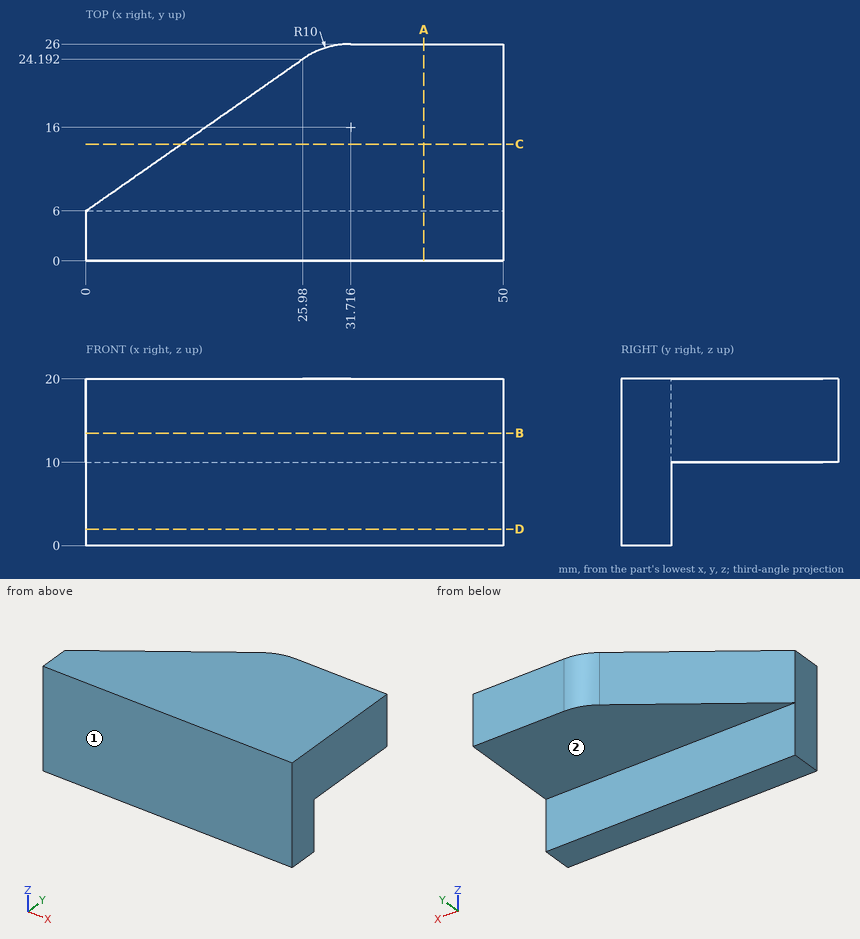
Input: dimensioned drawing with shaded views. Units: mm. Origin: part minimum x, y, z. A direction names the side the tool comes from. Coordinates: 2 decimals unless noted, no trailing zeros. Loops run counter-clockwise (first coordinate to the right, second up) from the corner with the lowest first, then second, coordinate; pieces in that order, holes last.
Q1. Set-up query: the marked faces 1 and 2. Return all of +Z, -Z, +X, -X, +Y, -Y with unobstructed straight access to the full face (end or side cutting, diameter ignored); none if empty.
Results are:
face 1: +Z, -Z, +X, -X, -Y
face 2: -Z, +X, -X, +Y
Q2. Section A-A, the plane x = 40.5. Return the cut outline in (y, z), and give its area (3 significant figures).
Results are:
outline: (0, 0) - (6, 0) - (6, 10) - (26, 10) - (26, 20) - (0, 20) - close
area: 320 mm2
Q3. Contact query for a flat-ended pin moving along its axis: pin 1 (1.5 mm diameter, centred on x = 15.5, z = 8, fed in from +Y). Output: stop coordinate, or through.
Results are:
pin 1: stops at y = 6
Q4. Line query: line 1 along Y through (x, z) = (43, 5.25); line 2 along Z through (x, y) = (19.5, 14.25); line 3 along X through (y, z) = (19.5, 10.5). Output: solid intervals per line, ascending.
Results are:
line 1: y = 0 to 6
line 2: z = 10 to 20
line 3: x = 19.28 to 50
Q5. Section D-D, the plane z = 2. Return the cut outline in (x, y), and give its area (3 significant figures).
Results are:
outline: (0, 0) - (50, 0) - (50, 6) - (0, 6) - close
area: 300 mm2
Q6. Section B-B, the plane z = 13.5. Return the cut outline in (x, y) (1 decimal), and give its area (3 significant figures).
Results are:
outline: (0, 0) - (50, 0) - (50, 26) - (31.7, 26) arc R10 ccw to (26, 24.2) - (0, 6) - close
area: 1,010 mm2
Q7. Section C-C, the plane y = 14. Return the cut outline in (x, z) (1 decimal).
Results are:
outline: (11.4, 10) - (50, 10) - (50, 20) - (11.4, 20) - close
